from build123d import *

# Parameters (mm, degrees)
POCKET_DEPTH          = 7
POLARPATTERN_COUNT    = 2
POCKET001_DEPTH       = 8
POLARPATTERN001_COUNT = 16
SKETCH003_R           = 2.6
POCKET002_DEPTH       = 15
CHAMFER_SIZE          = 0.4


with BuildPart() as part:
    # Sketch → Revolution (revolve)
    with BuildSketch(Plane.XZ):
        Polygon((0, 0), (17, 0), (17, 7), (9, 7), (9, 15), (0, 15), align=None)
    revolve(axis=Axis((0, 0, 0), (0, 0, 1)))

    # Sketch001 (on Face3 of Revolution) → Pocket (cut)
    with BuildSketch(Plane(origin=(0, 0, 7), x_dir=(-1, 0, 0), z_dir=(0, 0, 1))):
        with BuildLine():
            Line((0, 17), (17, 17))
            Line((17, 17), (17, -17))
            Line((17, -17), (0, -17))
            ThreePointArc((0, -17), (13, -4), (0, 9))
            Line((0, 17), (0, 9))
        make_face()
    pocket = extrude(amount=-POCKET_DEPTH, mode=Mode.SUBTRACT)

    # PolarPattern: Pocket ×2 about axis
    polarpattern_axis = Axis((0, 0, 7), (0, 0, 1))
    for i in range(1, POLARPATTERN_COUNT):
        add(pocket.rotate(polarpattern_axis, i * 360 / POLARPATTERN_COUNT), mode=Mode.SUBTRACT)

    # Sketch002 (on Face5 of Revolution) → Pocket001 (cut)
    with BuildSketch(Plane(origin=(0, 0, 15), x_dir=(-1, 0, 0), z_dir=(0, 0, 1))):
        Polygon((-1.25, 9), (1.25, 9), (0.75, 7.5), (0.5, 6.5), (-0.5, 6.5), (-0.75, 7.5), align=None)
    pocket001 = extrude(amount=-POCKET001_DEPTH, mode=Mode.SUBTRACT)

    # PolarPattern001: Pocket001 ×16 about axis
    polarpattern001_axis = Axis((0, 0, 15), (0, 0, 1))
    for i in range(1, POLARPATTERN001_COUNT):
        add(pocket001.rotate(polarpattern001_axis, i * 360 / POLARPATTERN001_COUNT), mode=Mode.SUBTRACT)

    # Sketch003 (on Face5 of Revolution) → Pocket002 (cut)
    with BuildSketch(Plane(origin=(0, 0, 15), x_dir=(-1, 0, 0), z_dir=(0, 0, 1))):
        Circle(SKETCH003_R)
    extrude(amount=-POCKET002_DEPTH, mode=Mode.SUBTRACT)

    # Chamfer
    chamfer_edges = [part.edges().sort_by_distance(p)[0] for p in [
        (-2.6, 0, 7.5),
        (2.6, 0, 15),
        (2.6, 0, 0),
    ]]
    chamfer(chamfer_edges, length=CHAMFER_SIZE)


solid = part.part
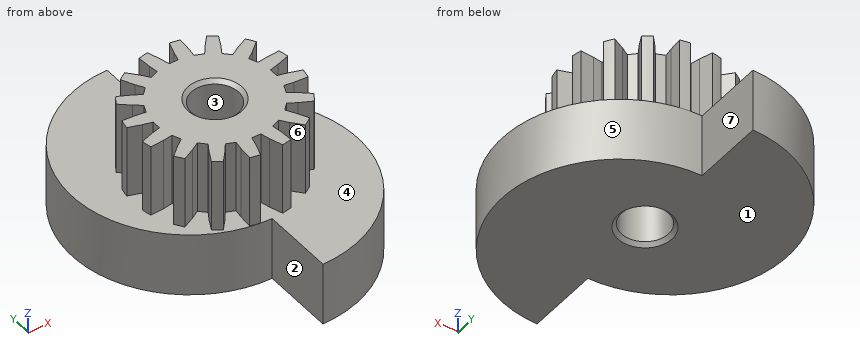
The listing builds one solid part. Answer for the finished solid, in the listing's coordinates (mm). Face numbers are marked on the shaded views. A direction names the side the tool comes from. Give positions to 0.01 mm unless a question says otherwise; leave off trailing zeros. Write each loop counter-clockwise with the first axis right and the second up, starting at its lowest first coordinate (ties: lowest second). Pieces come first, ordered by that corner, then holes.
1) Given P1, Ø1, axis at x = 7, z = 4.5, coming from the -Y side; P2, Ø7.5, axis at y = 13, z = 2, coming from the +X side; P3, Ø0.8, axis at y = 0, z = 9, coming from the +X side, each flat-ended and moving along its own axis, determine where each tip first touches the part or whether it passes through.
2) Section A-A (y = 0) is taken. Write down the section's boundary in (x, z), and give its area (3 significant figures).
3) A tool of negligible diameter and unlimited length cuts with its end or side. For the marked faces 4, 5, 6 and 7, from which of +Z, -Z, +X, -X, +Y, -Y can it reach the whole face along a straight path? Write none if from no direction.
4) For a pull along X with two mould halves and no side action, classify the marked faces 1, 2 and 3 as pulls with the +X half, pulls with the -X half, needs draft (parallel to the pull), parting line crosses it, or undercut.
5) Section C-C (x = -10.75) is taken. Write down the section's boundary in (y, z), and give its area (3 significant figures).
6) Find the intervals of material crossed by L1, parallel to X at y = 0, z = 7.25; L2, parallel to Y at x = 5, z = 11.75, in increasing order.
7) Section B-B (z = 5) is taken. Write down the section's boundary in (x, y), and give its area (3 significant figures).
Response:
1. P1: stops at y = -15.26
1. P2: stops at x = 0
1. P3: stops at x = 6.5
2. outline: (-12.37, 0) - (-3, 0) - (-2.6, 0.4) - (-2.6, 14.6) - (-3, 15) - (-6.5, 15) - (-6.5, 7) - (-12.37, 7) - close; (2.6, 0.4) - (3, 0) - (12.37, 0) - (12.37, 7) - (6.5, 7) - (6.5, 15) - (3, 15) - (2.6, 14.6) - close
2. area: 199 mm2
3. face 4: +Z
3. face 5: +Z, -Z, +X
3. face 6: +Z, -Y
3. face 7: +Z, -Z, +X, +Y
4. face 1: needs draft
4. face 2: pulls with the -X half
4. face 3: undercut
5. outline: (-3.31, 0) - (11.31, 0) - (11.31, 7) - (-3.31, 7) - close
5. area: 102 mm2
6. L1: x = -6.5 to -2.6, 2.6 to 6.5
6. L2: y = -7.48 to -6.29, -4.27 to 4.27, 6.29 to 7.48
7. outline: (0, -17) arc R13 ccw to (0, 9) - (0, 17) arc R13 ccw to (0, -9) - close; hole circle Ø5.2 at (0, 0)
7. area: 510 mm2
